Part print with two shaded views. Sizes in mm from the minimum x, y, z corner. Coordinates: 2 decimals unless noted, no trailing zeros. Loops run counter-clockwise (first coordinate to the right, second up) from the corner with the lowest first, then second, coordinate; pieces in that order, holes last. Notation, with made-up numbers: (4.25, 14) -> (43.25, 14) arc R36 cw to (43.25, 52) -> close; hole circle Ø7 at (66.25, -4). An arc over 180 degrees is marked (long way). One line per item, written item: value. Start each with the question number.
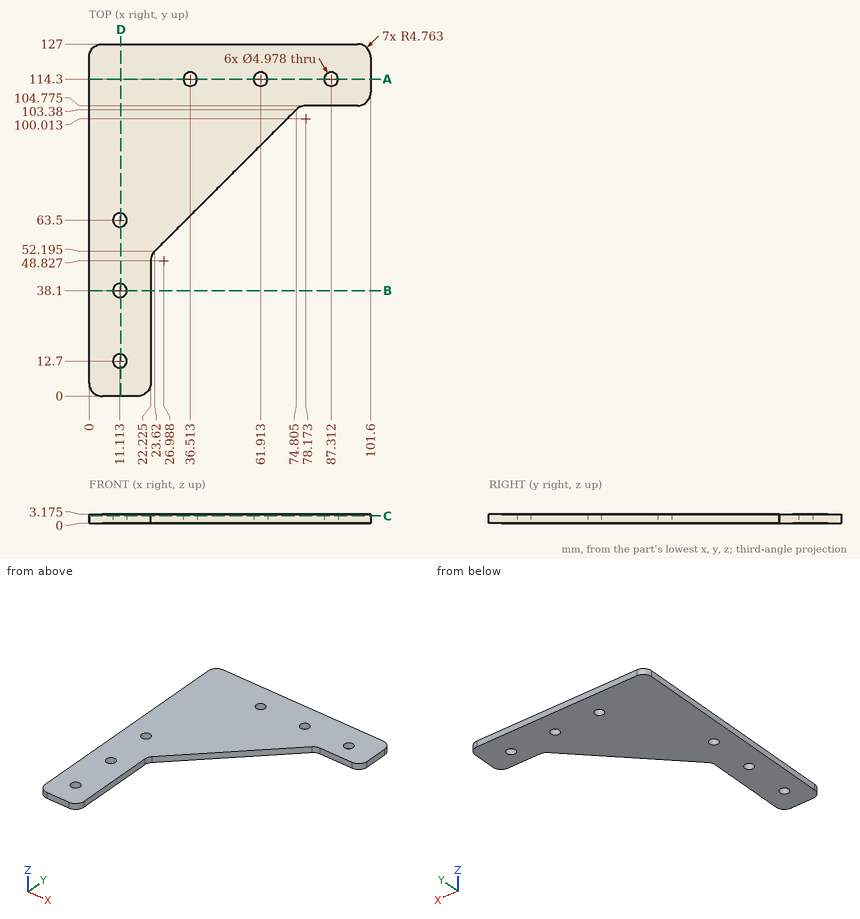
Item 1: Drop flat-ended pins along their axis: pin 1 Ø2 at (x, y) = (13, 32.5) entering from -Z; pin 2 Ø1 at (x, z) = (82.5, 3) entering from -Y (1 decimal); pin 3 Ø4.5 at (x, y) = (36.51, 114.3) entering from +Z. Give the stop position or say it passes through.
Item 2: Probe probe 1 along Y at (x, z) = (79, 1.1) (1 decimal); probe 2 along X at (y, z) = (88, 1) (1 decimal); probe 3 along Y at (x, z) = (35, 2.3) (1 decimal). List the from-to ranges inside material, lowest first.
Item 3: Band-saw the part on A-A, the plane y = 114.3. List the corners of the cut face in (x, z) (1 decimal), and give its area (3 significant figures).
Item 4: Band-saw the part on D-D, the plane x = 11.5. List the corners of the cut face in (y, z) (1 decimal).
Item 5: Band-saw the part on B-B, the plane y = 38.1. List the corners of the cut face in (x, z) (1 decimal).
Item 6: Band-saw the part on C-C, the plane z = 2.55. List the corners of the cut face in (x, y) (1 decimal).
Worked out:
1. pin 1: stops at z = 0
1. pin 2: stops at y = 104.8
1. pin 3: passes through
2. probe 1: y = 104.8 to 127
2. probe 2: x = 0 to 59.4
2. probe 3: y = 63.6 to 112.3, 116.3 to 127
3. outline: (0, 0) -> (34, 0) -> (34, 3.2) -> (0, 3.2) -> close; (39, 0) -> (59.4, 0) -> (59.4, 3.2) -> (39, 3.2) -> close; (64.4, 0) -> (84.8, 0) -> (84.8, 3.2) -> (64.4, 3.2) -> close; (89.8, 0) -> (101.6, 0) -> (101.6, 3.2) -> (89.8, 3.2) -> close
3. area: 275 mm²
4. outline: (0, 0) -> (10.2, 0) -> (10.2, 3.2) -> (0, 3.2) -> close; (15.2, 0) -> (35.6, 0) -> (35.6, 3.2) -> (15.2, 3.2) -> close; (40.6, 0) -> (61, 0) -> (61, 3.2) -> (40.6, 3.2) -> close; (66, 0) -> (127, 0) -> (127, 3.2) -> (66, 3.2) -> close
5. outline: (0, 0) -> (8.6, 0) -> (8.6, 3.2) -> (0, 3.2) -> close; (13.6, 0) -> (22.2, 0) -> (22.2, 3.2) -> (13.6, 3.2) -> close
6. outline: (0, 4.8) arc R4.8 ccw to (4.8, 0) -> (17.5, 0) arc R4.8 ccw to (22.2, 4.8) -> (22.2, 48.8) arc R4.8 cw to (23.6, 52.2) -> (74.8, 103.4) arc R4.8 cw to (78.2, 104.8) -> (96.8, 104.8) arc R4.8 ccw to (101.6, 109.5) -> (101.6, 122.2) arc R4.8 ccw to (96.8, 127) -> (4.8, 127) arc R4.8 ccw to (0, 122.2) -> close; hole circle Ø5 at (11.1, 12.7); hole circle Ø5 at (11.1, 38.1); hole circle Ø5 at (11.1, 63.5); hole circle Ø5 at (36.5, 114.3); hole circle Ø5 at (61.9, 114.3); hole circle Ø5 at (87.3, 114.3)
